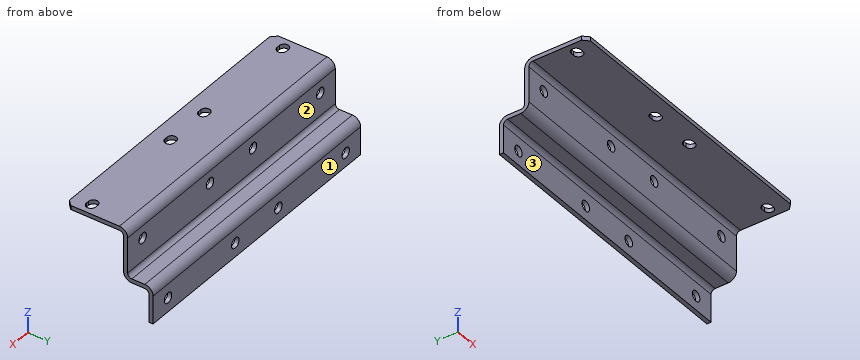
Autodesk Inventor part; units mm, degrees
ref_plane "YZ Plane" through (0, 0, 0) normal (1, 0, 0) x (0, 1, 0)
ref_plane "XZ Plane" through (0, 0, 0) normal (0, 1, 0) x (-1, 0, 0)
ref_plane "XY Plane" through (0, 0, 0) normal (0, 0, 1) x (1, 0, 0)
sketch "Sketch1" plane through (0, 0, 0) normal (0, 0, 1) x (1, 0, 0)
  line L0 (0, 0) -> (555, 0)
  line L1 (555, 0) -> (555, 120)
  line L2 (555, 120) -> (0, 120)
  line L3 (0, 120) -> (0, 0)
  dimension "d0" = 120
  dimension "d1" = 555
extrude "Plate1" add sketch "Sketch1" along normal blind 8
sketch "Sketch2" plane through (555, 112, 8) normal (0, 1, 0) x (-1, 0, 0)
  line L0 (555, 0) -> (0, 0)
  line L1 (0, 0) -> (0, -100)
  line L2 (0, -100) -> (555, -100)
  line L3 (555, -100) -> (555, 0)
edge flange "Flange1" height 100 angle 90 thickness 8 bend radius 8 thickness toward (0, 1, 0) relief tear relief width 8 relief depth 4 edges at (277.5, 120, 0) wall of the first edge with corners at (0, 112, 8) (555, 112, 8) (555, 112, -92) (0, 112, -92)
bend "Bend1"
corner "Corner1"
sketch "Sketch3" plane through (0, 112, -92) normal (0, -1, 0) x (1, 0, 0)
  line L0 (0, 0) -> (0, 84)
  line L1 (0, 0) -> (555, 0)
  line L2 (555, 0) -> (555, 84)
  circle A0 centre (40, 60) radius 10
  circle A1 centre (515, 60) radius 10
  circle A2 centre (220, 60) radius 10
  circle A3 centre (335, 60) radius 10
  point P0 (0, 92)
  dimension "d13" = 20
  dimension "d14" = 20
  dimension "d15" = 40
  dimension "d16" = 60
  dimension "d17" = 60
  dimension "d18" = 40
  dimension "d19" = 20
  dimension "d20" = 180
  dimension "d21" = 20
  dimension "d22" = 180
  dimension "d23" = 60
  dimension "d24" = 60
hole "Hole1" at (40, 112, -32) at (220, 112, -32) at (335, 112, -32) at (515, 112, -32) direction (0, 1, 0) diameter 20 depth 8 tip angle 118
sketch "Sketch4" plane through (0, 0, 8) normal (0, 0, 1) x (1, 0, 0)
  circle A0 centre (544.5, 10.5) radius 1.1625
  circle A1 centre (544.5, 59.5) radius 1.1625
  arc A2 (535.5, 26) -> (535.5, 44) centre (535.5, 35) ccw
  line L0 (535.5, 26) -> (529.5, 26)
  arc A3 (529.5, 44) -> (529.5, 26) centre (529.5, 35) ccw
  line L1 (529.5, 44) -> (535.5, 44)
  line L2 (507.5, 26.468) -> (507.5, 43.532)
  arc A4 (505.7408, 21) -> (507.5, 26.468) centre (471.6029, 35) ccw
  line L3 (505.7408, 21) -> (482.22, 0)
  line L4 (482.22, 0) -> (545, 0)
  line L5 (545, 0) -> (553, 8)
  line L6 (553, 8) -> (553, 62)
  line L7 (553, 62) -> (545, 70)
  line L8 (482.22, 70) -> (545, 70)
  line L9 (482.22, 70) -> (505.7408, 49)
  arc A5 (507.5, 43.532) -> (505.7408, 49) centre (471.6029, 35) ccw
  circle A6 centre (310.5, 10.5) radius 1.1625
  circle A7 centre (310.5, 59.5) radius 1.1625
  arc A8 (325.5, 26) -> (325.5, 44) centre (325.5, 35) ccw
  line L10 (325.5, 26) -> (319.5, 26)
  arc A9 (319.5, 44) -> (319.5, 26) centre (319.5, 35) ccw
  line L11 (319.5, 44) -> (325.5, 44)
  line L12 (347.5, 26.468) -> (347.5, 43.532)
  arc A10 (349.2592, 49) -> (347.5, 43.532) centre (383.3971, 35) ccw
  line L13 (349.2592, 49) -> (372.78, 70)
  line L14 (372.78, 70) -> (310, 70)
  line L15 (310, 70) -> (302, 62)
  line L16 (302, 8) -> (302, 62)
  line L17 (302, 8) -> (310, 0)
  line L18 (372.78, 0) -> (310, 0)
  line L19 (372.78, 0) -> (349.2592, 21)
  arc A11 (347.5, 26.468) -> (349.2592, 21) centre (383.3971, 35) ccw
  circle A12 centre (244.5, 10.5) radius 1.1625
  circle A13 centre (244.5, 59.5) radius 1.1625
  arc A14 (235.5, 26) -> (235.5, 44) centre (235.5, 35) ccw
  line L20 (235.5, 26) -> (229.5, 26)
  arc A15 (229.5, 44) -> (229.5, 26) centre (229.5, 35) ccw
  line L21 (229.5, 44) -> (235.5, 44)
  line L22 (207.5, 26.468) -> (207.5, 43.532)
  arc A16 (205.7408, 21) -> (207.5, 26.468) centre (171.6029, 35) ccw
  line L23 (205.7408, 21) -> (182.22, 0)
  line L24 (182.22, 0) -> (245, 0)
  line L25 (245, 0) -> (253, 8)
  line L26 (253, 8) -> (253, 62)
  line L27 (253, 62) -> (245, 70)
  line L28 (182.22, 70) -> (245, 70)
  line L29 (182.22, 70) -> (205.7408, 49)
  arc A17 (207.5, 43.532) -> (205.7408, 49) centre (171.6029, 35) ccw
  circle A18 centre (10.5, 10.5) radius 1.1625
  circle A19 centre (10.5, 59.5) radius 1.1625
  arc A20 (25.5, 26) -> (25.5, 44) centre (25.5, 35) ccw
  line L30 (25.5, 26) -> (19.5, 26)
  arc A21 (19.5, 44) -> (19.5, 26) centre (19.5, 35) ccw
  line L31 (19.5, 44) -> (25.5, 44)
  line L32 (47.5, 26.468) -> (47.5, 43.532)
  arc A22 (49.2592, 49) -> (47.5, 43.532) centre (83.3971, 35) ccw
  line L33 (49.2592, 49) -> (72.78, 70)
  line L34 (72.78, 70) -> (10, 70)
  line L35 (10, 70) -> (2, 62)
  line L36 (2, 8) -> (2, 62)
  line L37 (2, 8) -> (10, 0)
  line L38 (72.78, 0) -> (10, 0)
  line L39 (72.78, 0) -> (49.2592, 21)
  arc A23 (47.5, 26.468) -> (49.2592, 21) centre (83.3971, 35) ccw
extrude "Extrusion1" cut sketch "Sketch4" against normal blind 10 contours L0 A3 L1 A2 | L10 A9 L11 A8 | L20 A15 L21 A14 | L30 A21 L31 A20
chamfer "Corner Chamfer1" distance 10 angle 45 2 edges at (555, 0, 4) (0, 0, 4)
sketch "Sketch5" plane through (0, 112, -84) normal (0, 0, -1) x (-1, 0, 0)
  line L0 (-555, 0) -> (0, 0)
  line L1 (0, 0) -> (0, 57)
  line L2 (0, 57) -> (-555, 57)
  line L3 (-555, 57) -> (-555, 0)
edge flange "Flange2" height 57 angle 90 thickness 8 bend radius 8 thickness toward (0, 0, -1) relief tear relief width 8 relief depth 4 edges at (277.5, 120, -92) wall of the first edge with corners at (555, 112, -84) (0, 112, -84) (0, 169, -84) (555, 169, -84)
bend "Bend2"
corner "Corner2"
sketch "Sketch6" plane through (555, 161, -84) normal (0, 1, 0) x (-1, 0, 0)
  line L0 (555, 0) -> (0, 0)
  line L1 (0, 0) -> (0, -70)
  line L2 (0, -70) -> (555, -70)
  line L3 (555, -70) -> (555, 0)
edge flange "Flange3" height 70 angle 90 thickness 8 bend radius 8 thickness toward (0, 1, 0) relief tear relief width 8 relief depth 4 edges at (277.5, 169, -92) wall of the first edge with corners at (0, 161, -84) (555, 161, -84) (555, 161, -154) (0, 161, -154)
bend "Bend3"
corner "Corner3"
sketch "Sketch7" plane through (0, 161, -154) normal (0, -1, 0) x (1, 0, 0)
  line L0 (0, 0) -> (0, 54)
  line L1 (0, 0) -> (555, 0)
  line L2 (555, 0) -> (555, 54)
  circle A0 centre (40, 27) radius 10
  circle A1 centre (515, 27) radius 10
  circle A2 centre (220, 27) radius 10
  circle A3 centre (335, 27) radius 10
  point P0 (0, 154)
  dimension "d57" = 20
  dimension "d58" = 40
  dimension "d59" = 27
  dimension "d60" = 20
  dimension "d61" = 40
  dimension "d62" = 27
  dimension "d63" = 20
  dimension "d64" = 20
  dimension "d65" = 180
  dimension "d66" = 27
  dimension "d67" = 180
  dimension "d68" = 27
hole "Hole2" at (40, 161, -127) at (220, 161, -127) at (335, 161, -127) at (515, 161, -127) direction (0, 1, 0) diameter 20 depth 8 tip angle 118
equation "\"d30\" = Thickness"
equation "\"d74\" = Thickness"
equation "\"d3\" = BendReliefWidth"
equation "\"d4\" = BendReliefDepth"
equation "\"d5\" = MinimumRemnant"
equation "\"d6\" = BendRadius"
equation "\"d9\" = BendRadius"
equation "\"d10\" = CornerReliefSize"
equation "\"d11\" = GapSize"
equation "\"d12\" = JacobiRadiusSize"
equation "\"d37\" = BendReliefWidth"
equation "\"d38\" = BendReliefDepth"
equation "\"d39\" = MinimumRemnant"
equation "\"d40\" = BendRadius"
equation "\"d43\" = BendRadius"
equation "\"d44\" = CornerReliefSize"
equation "\"d45\" = GapSize"
equation "\"d46\" = JacobiRadiusSize"
equation "\"d47\" = BendReliefWidth"
equation "\"d48\" = BendReliefDepth"
equation "\"d49\" = MinimumRemnant"
equation "\"d50\" = BendRadius"
equation "\"d53\" = BendRadius"
equation "\"d54\" = CornerReliefSize"
equation "\"d55\" = GapSize"
equation "\"d56\" = JacobiRadiusSize"
equation "\"BendRadius\" = Thickness"
equation "\"BendReliefWidth\" = Thickness"
equation "\"BendReliefDepth\" = 0.5 * Thickness"
equation "\"CornerReliefSize\" = 4 * Thickness"
equation "\"MinimumRemnant\" = 2 * Thickness"
equation "\"TransitionRadius\" = BendRadius"
equation "\"JacobiRadiusSize\" = BendRadius"
equation "\"GapSize\" = Thickness"
equation "\"d2\" = BendRadius"
properties part number "Bearing Base"
Build history of the part. All positions in model axes, mm. Face numbers are marked on the shaded views. A direction names the side the tool comes from. Round coordinates to 2 decimals unless told otherwise and drop trailing zeros. Write each loop counter-clockwise with the first axis right and the second up, starting at its lowest first coordinate (ties: lowest second). Pieces come first, ordered by that corner, then holes. Notation, with made-up numbers: (75.5, -26) - (108.5, -26) arc R28 ccw to (108.5, -1) - close; hole circle Ø8 at (58.5, 55.25). An arc over 180 degrees is marked (long way). One line per question, with ' | ' between items.
1. Tool access for the marked faces 1, 2 and 3: list every direction of +Z, -Z, +X, -X, +Y, -Y with a clear straight run to the whole face (end or side of a thin tool).
Results are:
face 1: +Z, -Z, +X, -X, +Y | face 2: +Z, +X, -X, +Y | face 3: -Z, +X, -X, -Y
2. Band-saw the part on C-C, the plane y = 80. Write the cut outline in (x, z).
Results are:
outline: (0, 0) - (555, 0) - (555, 8) - (0, 8) - close
3. Band-saw the part on B-B, the plane x = 282.5. Write the cut outline in (y, z), and give its area (3 significant figures).
Results are:
outline: (0, 0) - (104, 0) arc R8 cw to (112, -8) - (112, -76) arc R16 ccw to (128, -92) - (153, -92) arc R8 cw to (161, -100) - (161, -154) - (169, -154) - (169, -100) arc R16 ccw to (153, -84) - (128, -84) arc R8 cw to (120, -76) - (120, -8) arc R16 ccw to (104, 8) - (0, 8) - close | area: 2,460 mm^2
4. Drill centre lines: line 1 along X through (y, z) = (164, -127); line 2 along Y through (x, z) = (136, -123.5); line 3 along Y through (x, z) = (141, -63.5). Where is each one in solid material? Low to high. Write a range as from..to.
Results are:
line 1: 0..30, 50..210, 230..325, 345..505, 525..555 | line 2: 161..169 | line 3: 112..120
5. Band-saw the part on A-A, the plane z = -127. Write the cut outline in (x, y), and give its area (3 significant figures).
Results are:
outline: (0, 161) - (30, 161) - (30, 169) - (0, 169) - close; (50, 161) - (210, 161) - (210, 169) - (50, 169) - close; (230, 161) - (325, 161) - (325, 169) - (230, 169) - close; (345, 161) - (505, 161) - (505, 169) - (345, 169) - close; (525, 161) - (555, 161) - (555, 169) - (525, 169) - close | area: 3,800 mm^2
6. Drop flat-ended pins along their axis: pin 1 Ø1.5 at (x, z) = (498, -53) entering from -Y; pin 2 Ø20 at (x, y) = (273.5, 139.5) entering from +Z; pin 3 Ø1.8 at (x, z) = (323.5, 2.5) entering from +Y; pin 4 Ø18 at (x, z) = (335, -127) entering from -Y. Give the stop position or say it passes through.
Results are:
pin 1: y = 112 | pin 2: z = -84 | pin 3: y = 116.8 | pin 4: through
